The listing builds one solid part. Answer for the finished solid, in the listing's coordinates (mm). A direction names the side the tool comes from. Coordinates: 2 decimals unless noted, no trailing zeros. Loops run counter-clockwise (first coordinate to the right, second up) from the corner with the lowest first, then second, coordinate; pieces in that order, holes last. Notation, with made-up numbers: (-19, -4.75) - (-9, -4.75) arc R23 ccw to (-9, 5.25) - close; hole circle Ø4 at (58, 38.25). An arc over 180 degrees is marked (long way). Write each question's results on one line, items separated by ' | '. Start each with the question number.
(1) Determine the mould class of faces 1 (the flat face through (37, 7.5, -109)), 2 (the cylindrical face through (-40.996, 0.76, -114.448)), 3 (the cylindrical face through (38.34, 4.46, -22.89)), 4 (the cylindrical face through (14.049, 0.74, -127.443)) for opening direction X: released by +X, released by -X, zero draft, split by the parting line, or undercut.
(2) Find section D-D on x = -20. Determine the outline of the cut face in (y, z), then the cut area to 3 significant figures.
(3) Given pin 1 Ø0.8 at (y, z) = (1, -85.5) entering from +X; pin 2 Ø1.2 at (y, z) = (0.5, -127) entering from -X; pin 3 Ø5 at (x, z) = (-23.5, -58) entering from +Y; pin 4 Ø2.5 at (x, z) = (-14.5, -128.87) entering from +Y, each flat-ended and moving along its own axis, determine where each tip first touches the part or whether it passes through.
(4) Find section C-C on z = -17. Determine the outline of the cut face in (x, y).
(5) For faces 5 (the cylindrical face through (-20.33, 4.46, -108.52)), 6 (the cylindrical face through (-31.425, 0.74, -85.614)), determine the directions among +Z, -Z, +X, -X, +Y, -Y from which every point of the face is accessible in a straight line to the end or side of a thin tool.
(6) Consider line 1 (X direction, y = 3, z = -25); line 2 (X direction, y = 0.65, z = -87); line 3 (Z direction, x = 37, y = 3.5). Determine where each line is inside the solid, lowest interval first. Write a range as from..to.
(7) Find section A-A on y = 3.25. Determine the outline of the cut face in (x, z).
(8) Find section B-B on x = 14.5. Determine the outline of the cut face in (y, z), then the cut area to 3 significant figures.
Autodesk Inventor part; units mm, degrees
sketch "Skizze1" plane through (0, 0, 0) normal (0, 1, 0) x (-1, 0, 0)
  line L0 (0, 0) -> (-52, 0)
  line L1 (-52, 0) -> (-52, -27)
  line L2 (-52, -27) -> (-42.5, -35.8741)
  line L3 (-42.5, -35.8741) -> (-42.5, -115.8741)
  line L4 (-42.5, -115.8741) -> (-26.5, -115.8741)
  line L5 (-26.5, -115.8741) -> (-26.5, -134.8741)
  line L6 (-26.5, -134.8741) -> (0, -134.8741)
  line L7 (0, -134.8741) -> (0, 0)
  dimension "d2" = 52
  dimension "d3" = 27
  dimension "d4" = 13
  dimension "d8" = 80
  dimension "d9" = 16
  dimension "d10" = 19
  dimension "d11" = 42.5
  dimension "d12" = 26.5
  dimension "d13" = 134.8741
extrude "Extrusion1" add sketch "Skizze1" along normal blind 1.5
fillet "Rundung1" radius 2 1 edges at (52, 0.75, 0)
fillet "Rundung2" radius 10 1 edges at (26.5, 0.75, -115.8741)
fillet "Rundung3" radius 5 1 edges at (42.5, 0.75, -115.8741)
fillet "Rundung4" radius 5 1 edges at (26.5, 0.75, -134.8741)
mirror "Spiegeln1" about plane through (0, 0, 0) normal (1, 0, 0) of "Extrusion1"
mirror "Spiegeln2" about plane through (0, 0, 0) normal (1, 0, 0) of "Rundung2", "Rundung4", "Rundung3", "Rundung1"
sketch "Skizze2" plane through (0, 1.5, 0) normal (0, 1, 0) x (1, 0, 0)
  line L0 (-26.5, 125.8741) -> (-26.5, 129.8741)
  line L1 (21.5, 134.8741) -> (-21.5, 134.8741)
  line L2 (26.5, 125.8741) -> (26.5, 129.8741)
  point P0 (0, 0)
  point P1 (14.5, 128.8741)
  point P2 (-14.5, 128.8741)
  dimension "d20" = 12
  dimension "d21" = 6
  dimension "d22" = 6
  dimension "d23" = 12
hole "Bohrung1" at (14.5, 1.5, -128.8741) at (-14.5, 1.5, -128.8741) direction (0, -1, 0) diameter 3 end through all
sketch "Skizze3" plane through (0, 1.5, 0) normal (0, 1, 0) x (1, 0, 0)
  line L0 (-52, 2) -> (-52, 27)
  line L1 (50, 0) -> (-50, 0)
  line L2 (52, 2) -> (52, 27)
  point P0 (0, 0)
  point P1 (32, 17)
  point P2 (-32, 17)
  point P3 (-32, 87)
  point P4 (32, 87)
  dimension "d31" = 20
  dimension "d32" = 17
  dimension "d33" = 20
  dimension "d34" = 17
  dimension "d42" = 70
  dimension "d43" = 70
  dimension "d44" = 20
  dimension "d45" = 20
hole "Bohrung3" at (32, 1.5, -17) at (-32, 1.5, -17) at (-32, 1.5, -87) at (32, 1.5, -87) direction (0, -1, 0) diameter 3 end through all
sketch "Skizze4" plane through (0, 1.5, 0) normal (0, 1, 0) x (1, 0, 0)
  circle A0 centre (37, 25) radius 2.5
  line L0 (50, 0) -> (-50, 0)
  line L1 (52, 2) -> (52, 27)
  circle A1 centre (37, 111) radius 2.5
  circle A2 centre (-20, 25) radius 2.5
  circle A3 centre (-20, 111) radius 2.5
  point P0 (0, 0)
  dimension "d53" = 5
  dimension "d54" = 25
  dimension "d55" = 15
  dimension "d56" = 5
  dimension "d57" = 86
  dimension "d58" = 15
  dimension "d59" = 5
  dimension "d60" = 25
  dimension "d61" = 57
  dimension "d62" = 5
  dimension "d63" = 57
  dimension "d64" = 86
extrude "Extrusion2" add sketch "Skizze4" along normal blind 6
sketch "Skizze5" plane through (-20, 7.5, -25) normal (0, 1, 0) x (1, 0, 0)
  circle A0 centre (57, 0) radius 2.5
  circle A1 centre (57, 86) radius 2.5
  circle A2 centre (0, 0) radius 2.5
  circle A3 centre (0, 86) radius 2.5
  point P0 (20, -25)
  dimension "d68" = 0
  dimension "d69" = 0
  dimension "d70" = 0
  dimension "d71" = 0
  dimension "d72" = 0
  dimension "d73" = 0
  dimension "d74" = 0
  dimension "d75" = 0
hole "Bohrung4" at (37, 7.5, -111) at (37, 7.5, -25) at (-20, 7.5, -25) at (-20, 7.5, -111) direction (0, -1, 0) diameter 3 end through all
thread "Gewinde1"
thread "Gewinde2"
thread "Gewinde3"
thread "Gewinde4"
ref_plane "Arbeitsebene1" through (0, 0, 0) normal (1, 0, 0) x (0, 1, 0)
properties part number "waveshare_expansion_board"
Values:
1) face 1: zero draft | face 2: released by -X | face 3: undercut | face 4: undercut
2) outline: (0, -134.87) - (1.5, -134.87) - (1.5, -113.5) - (7.5, -113.5) - (7.5, -112.5) - (0, -112.5) - close; (0, -109.5) - (7.5, -109.5) - (7.5, -108.5) - (1.5, -108.5) - (1.5, -27.5) - (7.5, -27.5) - (7.5, -26.5) - (0, -26.5) - close; (0, -23.5) - (7.5, -23.5) - (7.5, -22.5) - (1.5, -22.5) - (1.5, 0) - (0, 0) - close | area: 217 mm²
3) pin 1: stops at x = 42.5 | pin 2: stops at x = -26.5 | pin 3: stops at y = 1.5 | pin 4: passes through
4) outline: (-52, 0) - (-33.5, 0) - (-33.5, 1.5) - (-52, 1.5) - close; (-30.5, 0) - (30.5, 0) - (30.5, 1.5) - (-30.5, 1.5) - close; (33.5, 0) - (52, 0) - (52, 1.5) - (33.5, 1.5) - close
5) face 5: +Y | face 6: +Y, -Y
6) line 1: x = -22.5..-21.5, -18.5..-17.5, 34.5..35.5, 38.5..39.5 | line 2: x = -42.5..-33.5, -30.5..30.5, 33.5..42.5 | line 3: z = -113.5..-112.5, -109.5..-108.5, -27.5..-26.5, -23.5..-22.5
7) outline: circle Ø5 at (-20, -111); circle Ø5 at (-20, -25); circle Ø5 at (37, -111); circle Ø5 at (37, -25); hole circle Ø3 at (-20, -111); hole circle Ø3 at (-20, -25); hole circle Ø3 at (37, -111); hole circle Ø3 at (37, -25)
8) outline: (0, -134.87) - (1.5, -134.87) - (1.5, -130.37) - (0, -130.37) - close; (0, -127.37) - (1.5, -127.37) - (1.5, 0) - (0, 0) - close | area: 198 mm²
